Print and shaded views of the part. All mm, measured from the part's lowest x, y and z. A direction names the side the tool comes from. Coordinates: 2 decimals unless noted, no trailing zeros. Order: outer loops, then holes, each group sorted by start corner. A loop starts at its lowest first (then second) coordinate and runs counter-clockwise, first axis right, second up. Notation, with made-up numbers: (-30.75, 6) -> (9.25, 6) arc R21 cw to (9.25, 21) -> close; hole circle Ø6 at (73, -23.75). An arc over 180 degrees is marked (long way). Return JSON: item names as keys, results as strings. Group by question number.
1) Cut at A-A (z = 10). Write the cut outline in (x, y) (1 decimal), and give its area (4 significant figures).
2) Pull direction X, two halves, no side cores. Call the marked faces 3, 4, 5 and 6: +X half, -X half, draft (parallel to the pull), parting line (faces both ways), or undercut.
3) Cut at C-C (z = 80.4). Write the cut outline in (x, y) (1 decimal), and give its area (3 significant figures).
4) Cut at D-D (y = 8.5). Write the cut outline in (x, z) (1 decimal), and give its area (3 significant figures).
5) Cut at B-B (x = 13). Write the cut outline in (y, z), and give its area (3 significant figures).
6) Probe line 1 (X direction, y = 29, z = 68.5) (1 decimal); line 2 (Z direction, x = 30, y = 21.5); line 3 (Y direction, x = 52.5, z = 29.6) (1 decimal). List the from-to ranges inside material, lowest first.
7) Flat gauge pins, fed straight in: pin 1 (8 mm diameter, centred on x = 48, z = 64, fed in from -Y); pin 2 (2.5 mm diameter, centred on y = 17.5, z = 80.4, fed in from +X); pin 3 (17 mm diameter, centred on y = 17.5, z = 55, fed in from -X); pin 4 (17.5 mm diameter, centred on x = 24.5, y = 19, fed in from +Z). Where does each tip first touch, or does it go through?
8) Which spindle directions (+Z, -Z, +X, -X, +Y, -Y) get a long thin tool onto all of the face, cutting with end or side? Do the marked faces 1 and 2. Say none if no direction does.
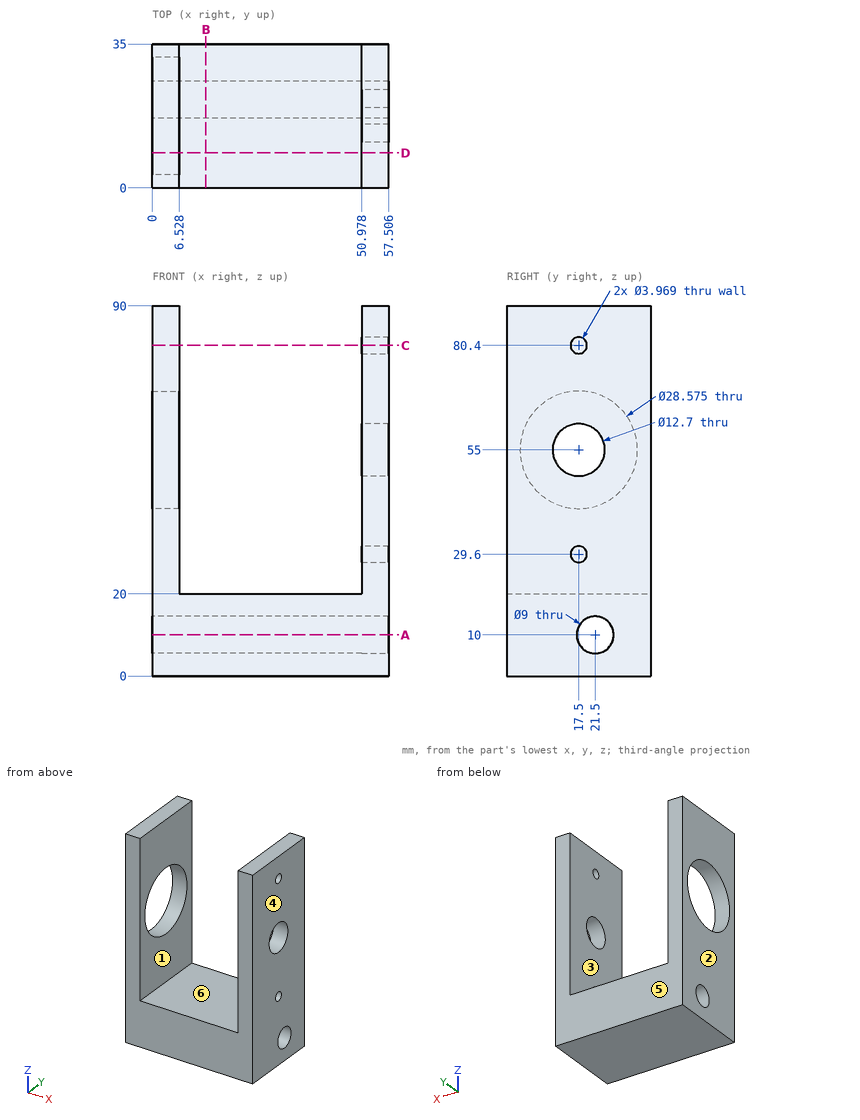
Answers below:
{
 "1": {"outline": "(0, 0) -> (57.5, 0) -> (57.5, 17) -> (0, 17) -> close; (0, 26) -> (57.5, 26) -> (57.5, 35) -> (0, 35) -> close", "area": "1,495 mm^2"},
 "2": {"face 3": "undercut", "face 4": "+X half", "face 5": "draft", "face 6": "undercut"},
 "3": {"outline": "(0, 0) -> (6.5, 0) -> (6.5, 35) -> (0, 35) -> close; (51, 0) -> (57.5, 0) -> (57.5, 15.5) -> (51, 15.5) -> close; (51, 19.5) -> (57.5, 19.5) -> (57.5, 35) -> (51, 35) -> close", "area": "431 mm^2"},
 "4": {"outline": "(0, 0) -> (57.5, 0) -> (57.5, 90) -> (51, 90) -> (51, 20) -> (6.5, 20) -> (6.5, 43.9) -> (0, 43.9) -> close; (0, 66.1) -> (6.5, 66.1) -> (6.5, 90) -> (0, 90) -> close", "area": "1,920 mm^2"},
 "5": {"outline": "(0, 0) -> (35, 0) -> (35, 20) -> (0, 20) -> close; hole circle Ø9 at (21.5, 10)", "area": "636 mm^2"},
 "6": {"line 1": "x = 0 to 6.5, 51 to 57.5", "line 2": "z = 0 to 5.5, 14.5 to 20", "line 3": "y = 0 to 15.5, 19.5 to 35"},
 "7": {"pin 1": "stops at y = 0", "pin 2": "stops at x = 6.53", "pin 3": "stops at x = 50.98", "pin 4": "stops at z = 20"},
 "8": {"face 1": "+Z, +Y, -Y", "face 2": "+Z, -Z, -X, +Y, -Y"}
}
